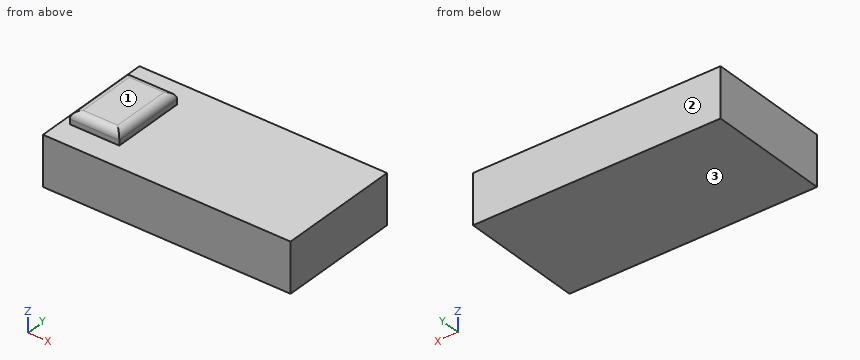
from build123d import *

# Parameters (mm, degrees)
F0_W     = 2000
F0_H     = 1000
F2_DEPTH = 400
F1_W     = 400
F1_H     = 600
F3_DEPTH = 100
F4_R     = 60


with BuildPart() as f2:
    # F0 (on Top) → F2 (new body)
    with BuildSketch(Plane.XY):
        with Locations((1.323093, -254.846548)):
            Rectangle(F0_W, F0_H)
    extrude(amount=-F2_DEPTH)

    # F1 (on face) → F3 (join)
    with BuildSketch(Plane.XY):
        with Locations((-738.085746, -254.846548)):
            Rectangle(F1_W, F1_H)
    extrude(amount=F3_DEPTH)

    # F4
    f4_edges = [f2.edges().sort_by_distance(p)[0] for p in [
        (-738.085746, -554.846548, 100),
        (-738.085746, 45.153452, 100),
        (-538.085746, -254.846548, 100),
        (-938.085746, -254.846548, 100),
    ]]
    fillet(f4_edges, radius=F4_R)


solid = f2.part
Input: part model. Units: mm. Frame: model coordinates. Face numbers are marked on the shaded views. Coordinates: 2 decimals unless noted, no trailing zeros. Loops run counter-clockwise (first coordinate to the right, second up) from the corner with the lowest first, then second, coordinate; pieces in that order, holes last. Notation, with made-up numbers: (-9, -14) -> (-1, -14) arc R32 ccw to (-1, 21) -> close; hole circle Ø8 at (0, 21.5). An arc over 180 degrees is marked (long way). Write each question's results on one line, items separated by ' | '. Start each with the question number.
Q1. Pin query (flat end, axial travel): pin 1 (8 mm diameter, centred on x = -545, y = -122.5, fed in from +Z); pin 2 (5 mm diameter, centred on x = -114.5, y = -118, fed in from +Z); pin 3 (5 mm diameter, centred on y = -110, z = 48, fed in from -X). Return the tip coordinate at first contact, or that it passes through.
Q2. Section D-D, the plane y = -669. Return the cut outline in (x, z), plus the area to 3 significant figures.
Q3. Section B-B, the plane y = -107. Return the cut outline in (x, z), plus the area to 3 significant figures.
Q4. Section C-C, the plane z = 65.5. Return the cut outline in (x, y).
Q5. Section A-A, the plane x = -792. Return the cut outline in (y, z).
Q6. Ray query, line 1 (X direction, y = -521.5, z = 21); line 2 (Z direction, x = 292, y = 143). Return the intervals inside material, ascending. Write a range as from..to.
Q7. Pull-direction query (Z, two-part tool) for the marked faces 1, 2 and 3; classes: released by +Z, released by -Z, zero draft, split by the parting line, or undercut.
Found:
1) pin 1: z = 74.5 | pin 2: z = 0 | pin 3: x = -937.83
2) outline: (-998.68, -400) -> (1001.32, -400) -> (1001.32, 0) -> (-998.68, 0) -> close | area: 800,000 mm2
3) outline: (-998.68, -400) -> (1001.32, -400) -> (1001.32, 0) -> (-538.09, 0) -> (-538.09, 40) arc R60 ccw to (-598.09, 100) -> (-878.09, 100) arc R60 ccw to (-938.09, 40) -> (-938.09, 0) -> (-998.68, 0) -> close | area: 838,000 mm2
4) outline: (-932.4, -549.16) -> (-543.77, -549.16) -> (-543.77, 39.47) -> (-932.4, 39.47) -> close
5) outline: (-754.85, -400) -> (245.15, -400) -> (245.15, 0) -> (45.15, 0) -> (45.15, 40) arc R60 ccw to (-14.85, 100) -> (-494.85, 100) arc R60 ccw to (-554.85, 40) -> (-554.85, 0) -> (-754.85, 0) -> close
6) line 1: -938.09..-538.09 | line 2: -400..0
7) face 1: released by +Z | face 2: zero draft | face 3: released by -Z
